The listing builds one solid part. Answer for the finished solid, in the listing's coordinates (mm). A direction names the side the tool comes from. Give positions to 0.01 mm unless a question says otherwise; leave off trailing zeros. Write each loop counter-clockwise with the first axis right and the second up, starting at its lowest first coordinate (ties: lowest second). Pieces come first, ordered by that corner, then holes. Notation, with made-up numbers: (18.25, 66.25) - (41.25, 66.25) arc R28 cw to (41.25, 91.25) - close; hole circle Ø2 at (8, -27.75). An arc over 180 degrees is marked (long way). Return JSON: item names as keys, results as strings.
from build123d import *

# Parameters (mm, degrees)
BOSS_EXTRUDE1_DEPTH = 1
SKETCH2_W           = 45
SKETCH2_H           = 14
BOSS_EXTRUDE2_DEPTH = 1
SKETCH3_W           = 1
SKETCH3_H           = 3
CUT_EXTRUDE1_DEPTH  = 1
FILLET1_R           = 0.5


with BuildPart() as part:
    # Sketch1 → Boss-Extrude1 (new body)
    with BuildSketch(Plane(origin=(0, 0, 0), x_dir=(1, 0, 0), z_dir=(0, 1, 0))):
        with BuildLine():
            Line((-20.5, -6), (20.5, -6))
            ThreePointArc((20.5, -6), (21.207106781, -5.707106781), (21.5, -5))
            Line((21.5, -5), (21.5, 5))
            ThreePointArc((21.5, 5), (21.207106781, 5.707106781), (20.5, 6))
            Line((20.5, 6), (-20.5, 6))
            ThreePointArc((-20.5, 6), (-21.207106781, 5.707106781), (-21.5, 5))
            Line((-21.5, 5), (-21.5, -5))
            ThreePointArc((-21.5, -5), (-21.207106781, -5.707106781), (-20.5, -6))
        make_face()
    extrude(amount=BOSS_EXTRUDE1_DEPTH)

    # Sketch2 → Boss-Extrude2 (add)
    with BuildSketch(Plane(origin=(0, 1, 0), x_dir=(1, 0, 0), z_dir=(0, 1, 0))):
        Rectangle(SKETCH2_W, SKETCH2_H)
    extrude(amount=BOSS_EXTRUDE2_DEPTH)

    # Sketch3 → Cut-Extrude1 (cut)
    with BuildSketch(Plane(origin=(0, 2, 0), x_dir=(1, 0, 0), z_dir=(0, 1, 0))):
        with Locations((22, 0)):
            Rectangle(SKETCH3_W, SKETCH3_H)
    extrude(amount=-CUT_EXTRUDE1_DEPTH, mode=Mode.SUBTRACT)

    # Fillet1
    fillet1_edges = [part.edges().sort_by_distance(p)[0] for p in [
        (21.5, 1.5, 1.5),
        (21.5, 1.5, -1.5),
    ]]
    fillet(fillet1_edges, radius=FILLET1_R)


solid = part.part
Item 1: A cutting plane is placed at B-B on z = -3.75. Determine the outline of the cut face in (x, y), then the cut area to 3 significant figures.
Answer below:
{"outline": "(-22.5, 1) - (-21.5, 1) - (-21.5, 0) - (21.5, 0) - (21.5, 1) - (22.5, 1) - (22.5, 2) - (-22.5, 2) - close", "area": "88.0 mm²"}
Item 2: A flat-ended cylindrical pin translates along its axis: P1, Ø0.5, axis at x = 5, y = 0.5, coming from the -Z side. Find the tip coordinate at first contact, or state that the pin passes through.
Answer below:
{"P1": "stops at z = -6"}
Item 3: Consider L1, parallel to Z at x = -2.5, y = 0.55; L2, parallel to X at y = 0.25, z = -1.25; L3, parallel to Y at x = -15, z = 6.25. Determine where each line is inside the solid, lowest interval first.
Answer below:
{"L1": "z = -6 to 6", "L2": "x = -21.5 to 21.5", "L3": "y = 1 to 2"}
Item 4: A cutting plane is placed at A-A on y = 0.55. Determine the outline of the cut face in (x, z), then the cut area to 3 significant figures.
Answer below:
{"outline": "(-21.5, -5) arc R1 ccw to (-20.5, -6) - (20.5, -6) arc R1 ccw to (21.5, -5) - (21.5, 5) arc R1 ccw to (20.5, 6) - (-20.5, 6) arc R1 ccw to (-21.5, 5) - close", "area": "515 mm²"}
Item 5: For faces 1 (the face through (-21.199, 0.493, -5.715)), 2 (the face through (21.199, 0.493, 5.715)), 3 (the face through (-21.215, 0.493, 5.699)), 4 (the face through (-1.8, 1, -6.3)), determine the directions among +Z, -Z, +X, -X, +Y, -Y from which every point of the face is accessible in a straight line to the end or side of a thin tool.
Answer below:
{"face 1": "-Z, -X, -Y", "face 2": "+Z, +X, -Y", "face 3": "+Z, -X, -Y", "face 4": "-Y"}
